from build123d import *

# Parameters (mm, degrees)
SKETCH_1_W              = 48
SKETCH_1_H              = 20
EXTRUDE_1_DEPTH         = 30
SKETCH_2_W              = 14
SKETCH_2_H              = 30
CUT_EXTRUDE_1_DEPTH     = 7
EXTRUDE_2_DEPTH         = 48
CUT_EXTRUDE_2_DEPTH     = 14
CUT_EXTRUDE_3_DEPTH     = 14
CUT_EXTRUDE_4_DEPTH     = 65.456478054
SKETCH_13_R             = 4
CUT_EXTRUDE_5_DEPTH     = 53.52066051
SKETCH_14_R             = 4
CUT_EXTRUDE_6_DEPTH     = 53.52066051
FILLET_1_R              = 7
EXTRUDE_5_DEPTH         = 1
SKETCH_20_R             = 7.5
CUT_EXTRUDE_8_DEPTH     = 53.52066051
BOSS_EXTRUDE1_DEPTH     = 25
CUT_EXTRUDE1_DEPTH      = 80.244164221
CUT_EXTRUDE1_DEPTH_BACK = 80.244164221


with BuildPart() as part:
    # Эскиз1 → Бобышка-Вытянуть1 (new body)
    with BuildSketch(Plane(origin=(0, 0, 0), x_dir=(1, 0, 0), z_dir=(0, 1, 0))):
        Rectangle(SKETCH_1_W, SKETCH_1_H)
    extrude(amount=EXTRUDE_1_DEPTH)

    # Эскиз2 → Вырез-Вытянуть1 (cut)
    with BuildSketch(Plane.XY.offset(10)):
        with Locations((0, 15)):
            Rectangle(SKETCH_2_W, SKETCH_2_H)
    extrude(amount=-CUT_EXTRUDE_1_DEPTH, mode=Mode.SUBTRACT)

    # Эскиз7 → Бобышка-Вытянуть2 (add)
    with BuildSketch(Plane(origin=(24, 0, 0), x_dir=(0, 0, -1), z_dir=(1, 0, 0))):
        Polygon((10, 0), (27.320508076, -10), (45.810889132, 22.026279442), (32, 30), (10, 30), align=None)
    extrude(amount=-EXTRUDE_2_DEPTH)

    # Эскиз8 → Вырез-Вытянуть2 (cut)
    with BuildSketch(Plane(origin=(24, 0, 0), x_dir=(0, 0, -1), z_dir=(1, 0, 0))):
        Polygon((10, 0), (10, 30), (32, 30), (45.810889132, 22.026279442), (27.320508076, -10), align=None)
    extrude(amount=-CUT_EXTRUDE_2_DEPTH, mode=Mode.SUBTRACT)

    # Эскиз9 → Вырез-Вытянуть3 (cut)
    with BuildSketch(Plane.ZY.offset(24)):
        Polygon((-10, 0), (-10, 30), (-32, 30), (-45.810889132, 22.026279442), (-27.320508076, -10), align=None)
    extrude(amount=-CUT_EXTRUDE_3_DEPTH, mode=Mode.SUBTRACT)

    # Эскиз11 → Вырез-Вытянуть4 (cut, through all)
    with BuildSketch(Plane.ZY.offset(10)):
        Polygon((-17.085266521, 5.482226936), (-27.285266521, 23.149145173), (-36.291930721, 17.949145173), (-26.091930721, 0.282226936), align=None)
    extrude(amount=-CUT_EXTRUDE_4_DEPTH, mode=Mode.SUBTRACT)

    # Эскиз13 → Вырез-Вытянуть5 (cut, through all)
    with BuildSketch(Plane(origin=(0, 0, -10), x_dir=(-1, 0, 0), z_dir=(0, 0, -1))):
        with Locations((17, 15)):
            Circle(SKETCH_13_R)
    extrude(amount=-CUT_EXTRUDE_5_DEPTH, mode=Mode.SUBTRACT)

    # Эскиз14 → Вырез-Вытянуть6 (cut, through all)
    with BuildSketch(Plane(origin=(0, 0, -10), x_dir=(-1, 0, 0), z_dir=(0, 0, -1))):
        with Locations((-17, 15)):
            Circle(SKETCH_14_R)
    extrude(amount=-CUT_EXTRUDE_6_DEPTH, mode=Mode.SUBTRACT)

    # Скругление1
    fillet_1_edges = [part.edges().sort_by_distance(p)[0] for p in [
        (-7, 15, 3),
        (7, 15, 3),
    ]]
    fillet(fillet_1_edges, radius=FILLET_1_R - 0.0001)  # a hair under: the kernel refuses the full size

    # Эскиз18 → Бобышка-Вытянуть5 (add)
    with BuildSketch(Plane(origin=(0, -14.330127019, -24.820508076), x_dir=(-1, 0, 0), z_dir=(0, -0.4999999999999885, -0.8660254037844454))):
        Polygon((2.153846154, 23.490381057), (2.153846154, 15.490381057), (1.025641026, 15.490381057), (1.025641026, 22.567304134), (-2.769230769, 22.567304134), (-2.769230769, 23.490381057), align=None)
    extrude(amount=EXTRUDE_5_DEPTH)

    # Эскиз20 → Вырез-Вытянуть8 (cut, through all)
    with BuildSketch(Plane(origin=(0, 0, -10), x_dir=(-1, 0, 0), z_dir=(0, 0, -1))):
        with Locations((-17, 15)):
            Circle(SKETCH_20_R)
        with Locations((17, 15)):
            Circle(SKETCH_20_R)
    extrude(amount=CUT_EXTRUDE_8_DEPTH, mode=Mode.SUBTRACT)

    # Sketch3 → Boss-Extrude1 (add)
    with BuildSketch(Plane(origin=(0, 30, 0), x_dir=(1, 0, 0), z_dir=(0, 1, 0))):
        with BuildLine():
            Line((7, -10), (24, -10))
            Line((24, -10), (24, 10))
            Line((24, 10), (10, 10))
            Line((10, 10), (10, 32))
            Line((10, 32), (-10, 32))
            Line((-10, 32), (-10, 10))
            Line((-10, 10), (-24, 10))
            Line((-24, 10), (-24, -10))
            Line((-24, -10), (-7, -10))
            ThreePointArc((-7, -10), (0, -3), (7, -10))
        make_face()
    extrude(amount=BOSS_EXTRUDE1_DEPTH)

    # Sketch4 → Cut-Extrude1 (cut, two sides: drawn at the far end of the back side and taken through both)
    with BuildSketch(Plane.ZY.offset(10).offset(-CUT_EXTRUDE1_DEPTH_BACK)):
        Polygon((-251.050138341, -96.468656337), (-45.810889132, 22.026279442), (35.63071017, 69.046608722), (240.869959379, 187.541544501), (3.880087821, 598.020042918), (-488.040009899, 314.00984208), align=None)
    extrude(amount=CUT_EXTRUDE1_DEPTH + CUT_EXTRUDE1_DEPTH_BACK, mode=Mode.SUBTRACT)


solid = part.part
Model file for the job. Use its own axes, mm. A direction names the side the tool comes from. Give positions to 0.01 mm unless a question says otherwise; leave off trailing zeros. Order: outer loops, then holes, each group sorted by start corner. A loop starts at its lowest first (then second) coordinate and runs counter-clockwise, first axis right, second up. Notation, with made-up numbers: (26, 25.5) - (82, 25.5) arc R37 cw to (82, 64.5) - close; hole circle Ø11 at (-24.75, -27). An arc over 180 degrees is marked (long way). One line per item, written item: value.
Item 1: Tool access for faces 1 (the flat face through (10, 27, -24)), 2 (the flat face through (-0.14, 9.239, -31.263)), 3 (the cylindrical face through (-4.9, 15.2, 5)): list every direction of +Z, -Z, +X, -X, +Y, -Y with a clear straight run to the whole face (end or side of a thin tool).
Response values:
face 1: -Z, +X, +Y, -Y
face 2: +X, -X
face 3: +Z, +Y, -Y
Item 2: Pin check, flat tips, straight feed: pin 1 Ø6 at (x, z) = (-7.5, -3.5) entering from -Y; pin 2 Ø8 at (x, y) = (16, 46) entering from -Z; pin 3 Ø20 at (y, z) = (24.5, -20.5) entering from +X. Stop position of each tip, or through.
Response values:
pin 1: y = 0
pin 2: z = -10
pin 3: x = 10
Item 3: Two-plate mould, pull along Y, no slides. Class faces 4 (the flat face through (-24, 27, 0)), 5 (the cylindrical face through (-9.5, 15, -17)), 6 (the flat face through (0.14, -4.93, -18.54)): released by +Y, released by -Y, zero draft, split by the parting line, or undercut.
Response values:
face 4: zero draft
face 5: undercut
face 6: released by -Y
Item 4: Slice it at C-C (y = 14). Give the number of separate pieces and of enclosed holes in the cut face, then the cut area to 3 significant figures.
Response values:
separate pieces: 4
enclosed holes: 0
area: 940 mm2
Item 5: Slice it at A-A (x = 8). List the corners of the cut face in (y, z), then the cut area to 3 significant figures.
Response values:
outline: (-10, -27.32) - (22.03, -45.81) - (54.25, 10) - (0, 10) - (0, -10) - close; hole (0.28, -26.09) - (17.95, -36.29) - (23.15, -27.29) - (5.48, -17.09) - close
area: 1,890 mm2
Item 6: Slice it at B-B (x = 17). List the corners of the cut face in (y, z).
Response values:
outline: (0, -10) - (11, -10) - (11, 10) - (0, 10) - close; (19, -10) - (42.7, -10) - (54.25, 10) - (19, 10) - close
Item 7: Wall check: line 1 (Z direction, x = -10, y = 12.5); line 2 (Z direction, x = -1, y = 18.5) (3 decimals); line 3 (Y direction, x = 17, z = -5.5). Give the ranges that are in metal, low to high.
Response values:
line 1: -10 to 10
line 2: -43.775 to -35.338, -24.601 to 3.072
line 3: 0 to 11, 19 to 45.3
